Read the model definition and answer for the solid it produces. Units are mm, in the model's axes. A direction names the side the tool comes from. Give positions to 0.01 mm unless a question says otherwise; leave off trailing zeros. Order: outer loops, then holes, each group sorted by start corner. A loop starts at its lowest first (then second) coordinate and runs counter-clockwise, first axis right, second up. Notation, with made-up numbers: (79, 48) -> (116, 48) arc R13 cw to (116, 68) -> close; hole circle Ø5 at (-31, -23.75). An arc over 180 degrees is marked (long way). Use one line per item in the form item = value.
Autodesk Inventor part; units mm, degrees
ref_plane "YZ Plane" through (0, 0, 0) normal (1, 0, 0) x (0, 1, 0)
ref_plane "XZ Plane" through (0, 0, 0) normal (0, 1, 0) x (-1, 0, 0)
ref_plane "XY Plane" through (0, 0, 0) normal (0, 0, 1) x (1, 0, 0)
sketch "Sketch1" plane through (0, 0, 0) normal (0, 0, 1) x (1, 0, 0)
  line L0 (23.85, 0) -> (46.0756, 0)
  line L1 (46.0756, 0) -> (46.0756, 12.7)
  line L2 (46.0756, 12.7) -> (0, 12.7)
  line L3 (0, 12.7) -> (0, 0)
  line L4 (17.5514, 12.7) -> (17.5514, -2.5)
  line L5 (46.0756, 8.9662) -> (42.3672, 8.9662)
  line L6 (42.3672, 7.747) -> (42.3672, 0)
  line L7 (46.0756, 7.747) -> (42.3672, 7.747)
  line L8 (46.0756, 8.9662) -> (42.3672, 7.747)
  line L9 (0, 11.1252) -> (0, 12.7)
  line L10 (17.5514, 0) -> (23.85, 0)
  line L11 (23.85, 0) -> (23.85, -2.5)
  line L12 (23.85, -2.5) -> (0, -2.5)
  line L13 (0, -2.5) -> (0, 0)
  dimension "d0" = 46.0756
  dimension "d1" = 12.7
  dimension "d2" = 17.5514
  dimension "d3" = 3.7338
  dimension "d4" = 42.3672
  dimension "d6" = 4.953
  dimension "d14" = 23.85
  dimension "d15" = 2.5
revolve "Revolution1" add sketch "Sketch1" angle 360 about axis through (0, 12.7, 0) along (0, -1, 0) contours L10 L4 L2 L1 L8 L6 L0 | L11 L12 L4 L10
sketch "Sketch2" plane through (0, 12.7, 0) normal (0, 1, 0) x (1, 0, 0)
  circle A0 centre (0, 0) radius 38.1
  dimension "d11" = 76.2
extrude "Extrusion1" cut sketch "Sketch2" against normal blind 1.5748
sketch "Sketch4" plane through (0, 11.1252, 0) normal (0, 1, 0) x (1, 0, 0)
  circle A0 centre (0, 0) radius 30.1752
  line L0 (-11.5475, 27.8782) -> (11.5475, -27.8782)
  circle A1 centre (0, 0) radius 17.5514
  line L1 (0, 0) -> (0, -30.1752)
  circle A2 centre (30.1752, 0) radius 3.2512
  circle A3 centre (-30.1752, 0) radius 1.7018
  dimension "d25" = 60.3504
  dimension "d27" = 22.5
hole "Hole2" at (-11.5475, 11.1252, -27.8782) at (11.5475, 11.1252, 27.8782) at (30.1752, 11.1252, 0) at (-30.1752, 11.1252, 0) direction (0, -1, 0) diameter 3.4036 end through all counterbore diameter 6.5024 counterbore depth 3.4036
sketch "Sketch5" plane through (0, 11.1252, 0) normal (0, 1, 0) x (1, 0, 0)
  circle A0 centre (0, 0) radius 30.1752
  point P0 (0, 30.1752)
  point P1 (0, -30.1752)
  dimension "d35" = 60.3504
hole "Hole3" at (0, 11.1252, -30.1752) at (0, 11.1252, 30.1752) direction (0, -1, 0) diameter 6.35 depth 7.62
fillet "Fillet1" radius 3.175 1 edges at (-42.3672, 0, 0)
properties part number "2016.06.09 Mount Adapter"
Item 1: The part is cut by section C-C on z = 0. State how many separate pieces and enclosed holes the cut face has, and give its area (3 significant figures).
Checks:
separate_pieces = 4
enclosed_holes = 0
area = 528 mm²
Item 2: Straight lines are drawn through the part: L1, parallel to Z at x = 2.5, y = 4.5; L2, parallel to X at y = 10.5, z = -2; L3, parallel to Y at x = -38.5, z = -1.5. For each, find the intervals that lie inside material, in ascending order. Write a range as from..to.
Checks:
L1 = -42.29..-32.13, -28.22..-17.37, 17.37..28.22, 32.13..42.29
L2 = -46.03..-32.74, -27.61..-17.44, 17.44..27.61, 32.74..46.03
L3 = 0..12.7
Item 3: Which of the six approach directions +Z, -Z, +X, -X, +Y, -Y give full straight-line access (tool end or side, diameter ignored) to faces 1 (the flat face through (17, 0, -17)), 2 (the flat face through (0, 3.505, -30)), 3 (the cylindrical face through (12.2, 3.81, 29.45))?
Checks:
face_1 = -Y
face_2 = +Y
face_3 = +Y, -Y
Item 4: Determine the mould class of faces 4 (the flat face through (12.9, 7.722, 29.3)), 5 (the conical face through (-9.235, 7.823, 41.586)), 6 (the flat face through (-2, -2.5, 18)) for opening direction Z: +Z half, -Z half, draft (parallel to the pull), parting line (faces both ways), or undercut.
Checks:
face_4 = undercut
face_5 = parting line
face_6 = draft
Item 5: Given pin 1 Ø7 at (x, z) = (28.5, -1) entering from +Y; pin 2 Ø5 at (y, z) = (8.5, 16.5) entering from +X; pin 3 Ø6 at (x, z) = (-30.18, 0) entering from +Y, each flat-ended and moving along its own axis, determine where each tip first touches the part or whether it passes through.
Checks:
pin_1 = 11.13
pin_2 = 43.88
pin_3 = 7.72
Item 6: The part is cut by section B-B on y = 1.75. Give the vertices of the cut face in (x, z), and give its area (3 significant figures).
Checks:
outline = circle Ø84.06 at (0, 0); hole circle Ø3.4 at (-30.18, 0); hole circle Ø35.1 at (0, 0); hole circle Ø3.4 at (-11.55, -27.88); hole circle Ø3.4 at (11.55, 27.88); hole circle Ø3.4 at (30.18, 0)
area = 4,550 mm²
